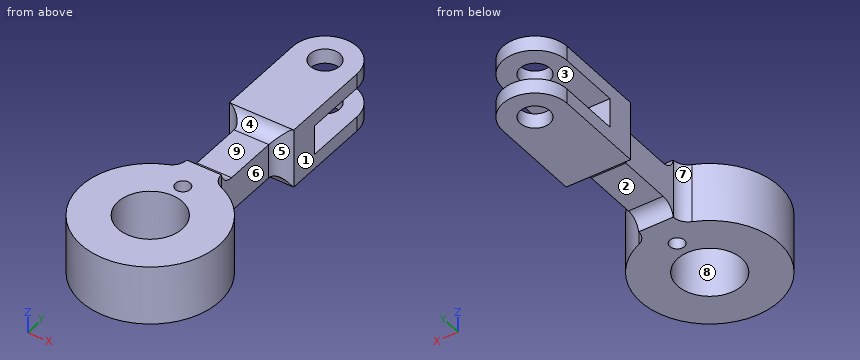
from build123d import *

# Parameters (mm, degrees)
SKETCH1_R               = 6.5
SKETCH1_R_2             = 1.5
SKETCH1_R_3             = 3
BOSS_EXTRUDE1_DEPTH     = 6
CUT_EXTRUDE1_DEPTH      = 60.483190903
CUT_EXTRUDE1_DEPTH_BACK = 60.483190903
SKETCH2_W               = 6
SKETCH2_H               = 19


with BuildPart() as part:
    # Sketch1 → Boss-Extrude1 (new, symmetric)
    with BuildSketch(Plane.XY):
        with BuildLine():
            Line((-3.5, 15.708278072), (-3.5, 29.5))
            ThreePointArc((-3.5, 29.5), (-4.378679656, 31.621320344), (-6.5, 32.5))
            Line((-6.5, 32.5), (-6.5, 51))
            ThreePointArc((-6.5, 51), (0, 57.5), (6.5, 51))
            Line((6.5, 51), (6.5, 32.5))
            ThreePointArc((6.5, 32.5), (4.378679656, 31.621320344), (3.5, 29.5))
            Line((3.5, 29.5), (3.5, 15.708278072))
            ThreePointArc((3.5, 15.708278072), (4.00588929, 14.041121282), (5.352941176, 12.936229001))
            ThreePointArc((5.352941176, 12.936229001), (0, -14), (-5.352941176, 12.936229001))
            ThreePointArc((-5.352941176, 12.936229001), (-4.00588929, 14.041121282), (-3.5, 15.708278072))
        make_face()
        Circle(SKETCH1_R, mode=Mode.SUBTRACT)
        with Locations((0, 9.5)):
            Circle(SKETCH1_R_2, mode=Mode.SUBTRACT)
        with Locations((0, 51)):
            Circle(SKETCH1_R_3, mode=Mode.SUBTRACT)
    extrude(amount=BOSS_EXTRUDE1_DEPTH, both=True)

    # Sketch2 → Cut-Extrude1 (cut, two sides: drawn at the far end of the back side and taken through both)
    with BuildSketch(Plane(origin=(0, 0, 0), x_dir=(0, 0, -1), z_dir=(1, 0, 0)).offset(-CUT_EXTRUDE1_DEPTH_BACK)):
        with BuildLine():
            Line((-6, 32.5), (-6, 15.708278072))
            ThreePointArc((-6, 15.708278072), (-4.208712153, 16.729826291), (-3.5, 18.666317964))
            Line((-3.5, 18.666317964), (-3.5, 29.541960108))
            ThreePointArc((-3.5, 29.541960108), (-4.208712153, 31.478451782), (-6, 32.5))
        make_face()
        with BuildLine():
            Line((6, 32.5), (6, 15.708278072))
            ThreePointArc((6, 15.708278072), (4.208712153, 16.729826291), (3.5, 18.666317964))
            Line((3.5, 18.666317964), (3.5, 29.541960108))
            ThreePointArc((3.5, 29.541960108), (4.208712153, 31.478451782), (6, 32.5))
        make_face()
        with Locations((0, 48)):
            Rectangle(SKETCH2_W, SKETCH2_H)
    extrude(amount=CUT_EXTRUDE1_DEPTH + CUT_EXTRUDE1_DEPTH_BACK, mode=Mode.SUBTRACT)


solid = part.part
The model under review builds one solid part; all positions refer to its coordinate system, in mm. Face numbers are marked on the shaded views. A direction names the side the tool comes from. Round coordinates to 2 decimals unless told otherwise and drop trailing zeros. Loops run counter-clockwise (first coordinate to the right, second up) from the corner with the lowest first, then second, coordinate; pieces in that order, holes last. Notation, with made-up numbers: (2.25, -15.75) -> (31.25, -15.75) arc R22 ccw to (31.25, -0.75) -> close; hole circle Ø10 at (-12.5, 30). An arc over 180 degrees is marked (long way). One line per question, with ' | ' between items. Start each with the question number.
Item 1: Draft analysis for pull direction X (two halves, no side actions). For the marked faces 6, 7, 8 and 9, state which applies: +X half, -X half, draft (parallel to the pull), parting line (faces both ways), or undercut.
Item 2: Add section C-C, the plane x = 0. Count the separate pieces of the cut face and the enclosed holes in it, then the cut area to 3 significant figures.
Item 3: Add section A-A, the plane z = -1.75. Write out the cut boundary in (x, y), then the cut area to 3 significant figures.
Item 4: Add section D-D, the plane x = -4.25. Write out the cut boundary in (y, z).
Item 5: For pin 1 (6 mm diameter, centred on x = -11, z = 0.5, fed in from -Y); pin 2 (2 mm diameter, centred on x = -4, z = 4.5, fed in from -Y); pin 3 (1 mm diameter, centred on x = 10.5, z = 3, fed in from +Y), all flat-tipped, find the tip position at first contact; note any pin that passes through.
Item 6: Add section B-B, the plane y = 0. Write out the cut boundary in (x, z), then the cut area to 3 significant figures.
Item 7: Wall thickness on line 1 along Y through (x, z) = (6, -0.75); line 2 along Y through (x, z) = (5, -1.75); line 3 along Z through (x, y) = (-5, 50.5): over which ranges is each line inside the solid? List them lowest first. Write a range as [from, to].
Item 8: Machinability: for the marked faces 1, 2, 3, 4 and 5, which of the approach directions +Z, -Z, +X, -X, +Y, -Y give a long, thin tool a straight path to every point of the face, cutting with its end or side? Answer none if there is none.
Return value:
1) face 6: +X half | face 7: -X half | face 8: undercut | face 9: draft
2) separate pieces: 5 | enclosed holes: 0 | area: 439 mm2
3) outline: (-6.5, 32.5) arc R3 cw to (-3.5, 29.5) -> (-3.5, 15.71) arc R3 cw to (-5.35, 12.94) arc R14 ccw (long way) to (5.35, 12.94) arc R3 cw to (3.5, 15.71) -> (3.5, 29.5) arc R3 cw to (6.5, 32.5) -> (6.5, 38.5) -> (-6.5, 38.5) -> close; hole circle Ø13 at (0, 0); hole circle Ø3 at (0, 9.5) | area: 690 mm2
4) outline: (-13.34, -6) -> (-4.92, -6) -> (-4.92, 6) -> (-13.34, 6) -> close; (4.92, -6) -> (13.72, -6) -> (13.72, 6) -> (4.92, 6) -> close; (31.48, -4.21) arc R3 cw to (32.5, -6) -> (55.92, -6) -> (55.92, -3) -> (38.5, -3) -> (38.5, 3) -> (55.92, 3) -> (55.92, 6) -> (32.5, 6) arc R3 cw to (31.48, 4.21) -> close
5) pin 1: stops at y = -11.49 | pin 2: stops at y = -13.67 | pin 3: stops at y = 9.8
6) outline: (-14, -6) -> (-6.5, -6) -> (-6.5, 6) -> (-14, 6) -> close; (6.5, -6) -> (14, -6) -> (14, 6) -> (6.5, 6) -> close | area: 180 mm2
7) line 1: y = [-12.65, -2.5], [2.5, 12.65], [32.46, 38.5] | line 2: y = [-13.08, -4.15], [4.15, 13.11], [32.1, 38.5] | line 3: z = [-6, -3], [3, 6]
8) face 1: +Z, -Z, +X, +Y | face 2: -Z, +X, -X | face 3: +X, -X, +Y | face 4: +Z, +X, -X | face 5: +Z, -Z, +X
